Input: part model. Units: mm. Frame: model coordinates. Face numbers are marked on the shaded views. Round coordinates to 2 decimals unless told otherwise and drop trailing zeros. Loops run counter-clockwise (first coordinate to the right, second up) from the corner with the lowest first, then second, coordinate; pieces in that order, holes last. Notation, with made-up numbers: (72, 19) - (110, 19) arc R26 ccw to (110, 55) - close; hole circle Ø3 at (12, 41). An arc over 180 degrees is marked (long way). Use CSV: the item, a comma, the result in double quotes. Start each with the question number.
1. Cut plane C-C (y = 1.5). Return loops of the section in (x, z).
2. Material intervals for probe 1 along Z at (x, y) = (0, -0.25); probe 2 along X at (y, z) = (-1.5, 55); probe 3 along X at (y, z) = (0.5, 55), sorted ascending. Write a range as from..to.
3. Pull-direction query (Z, two-part tool) for the marked faces 1, 2, 3 and 4; classes: +Z half, -Z half, draft (parallel to the pull), parting line (faces both ways), or undercut.
4. Cut plane B-B (x = 0). Return loops of the section in (y, z) (3 decimals).
5. Pin query (flat end, axial travel): P1, Ø1.5, axis at y = 0.5, z = 50, coming from the -X side. Return the tip coordinate at first contact, or that it passes through.
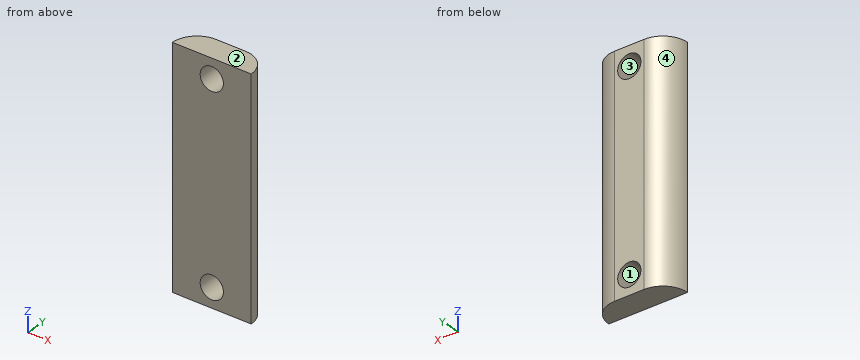
Autodesk Inventor part; units mm, degrees
ref_plane "YZ Plane" through (0, 0, 0) normal (1, 0, 0) x (0, 1, 0)
ref_plane "XZ Plane" through (0, 0, 0) normal (0, 1, 0) x (-1, 0, 0)
ref_plane "XY Plane" through (0, 0, 0) normal (0, 0, 1) x (1, 0, 0)
sketch "Sketch1" plane through (0, 0, 0) normal (0, 0, 1) x (1, 0, 0)
  line L0 (-10.16, 3.175) -> (10.16, 3.175)
  line L1 (10.16, 3.175) -> (10.16, -3.175)
  line L2 (10.16, -3.175) -> (-10.16, -3.175)
  line L3 (-10.16, -3.175) -> (-10.16, 3.175)
  line L4 (-10.16, 3.175) -> (10.16, -3.175) construction
  line L5 (10.16, 3.175) -> (-10.16, -3.175) construction
  point P0 (0, 0)
  dimension "d0" = 20.32
  dimension "d1" = 6.35
extrude "Extrusion1" add sketch "Sketch1" along normal blind 60
fillet "Fillet1" radius 6.35 2 edges at (-10.16, 3.175, 30) (10.16, 3.175, 30)
sketch "Sketch2" plane through (-3.81, 3.175, 0) normal (0, 1, 0) x (1, 0, 0)
  circle A0 centre (3.81, -5) radius 3
  line L0 (7.62, 0) -> (7.62, -60)
  circle A1 centre (3.81, -55) radius 3
  line L1 (7.62, -60) -> (0, -60)
  point P0 (3.81, 0)
  dimension "d5" = 6
  dimension "d6" = 5
  dimension "d7" = 3.81
  dimension "d10" = 6
  dimension "d11" = 3.81
  dimension "d15" = 50
extrude "Extrusion3" cut sketch "Sketch2" against normal through all
properties part number "Festoon_LowerBracket"
Established:
1,outline,"(-8.11, 0) - (8.11, 0) - (8.11, 60) - (-8.11, 60) - close; hole circle Ø6 at (0, 5); hole circle Ø6 at (0, 55)"
2,probe 1,"z = 0..2, 8..52, 58..60"
2,probe 2,"x = -9.94..-3, 3..9.94"
2,probe 3,"x = -8.99..-3, 3..8.99"
3,face 1,"undercut"
3,face 2,"+Z half"
3,face 3,"undercut"
3,face 4,"draft"
4,outline,"(-3.175, 0) - (3.175, 0) - (3.175, 2) - (-3.175, 2) - close; (-3.175, 8) - (3.175, 8) - (3.175, 52) - (-3.175, 52) - close; (-3.175, 58) - (3.175, 58) - (3.175, 60) - (-3.175, 60) - close"
5,P1,"stops at x = -9.45"
